from build123d import *

# Parameters (mm, degrees)
F1_DEPTH = 190.5
F2_W     = 260.35
F2_H     = 63.5
F3_DEPTH = 95.25
F4_W     = 31.75
F4_H     = 9.525
F4_R     = 3.175
F5_DEPTH = 76.2


with BuildPart() as f1:
    # F0 (on Right) → F1 (new body, symmetric)
    with BuildSketch(Plane.YZ):
        Polygon((-266.7, 25.4), (-266.7, 0), (0, 0), (0, 304.8), (-9.525, 304.8), (-9.525, 25.4), align=None)
    extrude(amount=F1_DEPTH, both=True)

    # F2 (on face) → F3 (join)
    with BuildSketch(Plane(origin=(0, 0, 0), x_dir=(-1, 0, 0), z_dir=(0, 1, 0))):
        with Locations((0, 31.75)):
            Rectangle(F2_W, F2_H)
    extrude(amount=F3_DEPTH)

    # F4 (on face) → F5 (join)
    with BuildSketch(Plane(origin=(0, 95.25, 0), x_dir=(-1, 0, 0), z_dir=(0, 1, 0))):
        with Locations((15.875, 14.2875)):
            Rectangle(F4_W, F4_H)
        with Locations((73.025, 14.2875)):
            Rectangle(F4_W, F4_H)
        with Locations((15.875, 33.3375)):
            Rectangle(F4_W, F4_H)
        with Locations((44.45, 14.2875)):
            Circle(F4_R)
    extrude(amount=F5_DEPTH)


solid = f1.part
Check sheet for the modelled part. Datum: model origin and axes. Units: mm. A direction names the side the tool comes from. Give positions to 0.01 mm unless a question says otherwise; leave off trailing zeros. Write each loop counter-clockwise with the first axis right and the second up, starting at its lowest first coordinate (ties: lowest second). Pieces come first, ordered by that corner, then holes. Notation, with made-up numbers: (35.5, -14) -> (51.5, -14) arc R14 cw to (51.5, -1) -> close; hole circle Ø7 at (-4.75, 2.5). An arc over 180 degrees is marked (long way). One line per item, written item: value. Start each with the question number.
Item 1: Section check A-A on x = 135.5. Record the cut outline in (y, z) (3 decimals).
Item 2: Section check D-D on z = 103. Record the cut outline in (x, y) (3 decimals).
Item 3: Section check B-B on y = 120. State how many separate pieces and enclosed holes the cut face has, then the cut area to 3 significant figures.
Item 4: Gauge pin test, flat ends, axial feed: pin 1 (12 mm diameter, centred on x = 129, z = 116, fed in from +Y); pin 2 (9.5 mm diameter, centred on x = -18, y = 138.5, fed in from +Z); pin 3 (4 mm diameter, centred on x = -7.5, z = 151, fed in from -Y) (3 decimals). Record the tip position at first contact, or that the pin passes through.
Item 5: Tool access check on faces 1 (the flat face through (130.175, 47, 31)), 2 (the flat face through (-16, 133, 19.05)), 3 (the flat face through (-130.175, 47, 31)), 4 (the flat face through (-73, 133, 19.05)). Record the directions out of +Z, -Z, +X, -X, +Y, -Y that give a thin tool (end or side, any length) a straight path to the whole face; none if there is none.
Item 6: Section check C-C on y = -32. Record the cut outline in (x, z).
Item 7: Material ranges on probe 1 along Z at (x, y) = (83, -48.5); probe 2 along Y at (x, z) = (-94, 129.5) (3 decimals); probe 3 along Z at (x, y) = (87, 21), recorded low to high. Write a range as from..to.
Results list:
1. outline: (-266.7, 0) -> (0, 0) -> (0, 304.8) -> (-9.525, 304.8) -> (-9.525, 25.4) -> (-266.7, 25.4) -> close
2. outline: (-190.5, -9.525) -> (190.5, -9.525) -> (190.5, 0) -> (-190.5, 0) -> close
3. separate pieces: 4
3. enclosed holes: 0
3. area: 939 mm²
4. pin 1: y = 0
4. pin 2: z = 38.1
4. pin 3: y = -9.525
5. face 1: +Z, -Z, +X, +Y
5. face 2: +X, -X, +Y
5. face 3: +Z, -Z, -X, +Y
5. face 4: +Z, +X, -X, +Y
6. outline: (-190.5, 0) -> (190.5, 0) -> (190.5, 25.4) -> (-190.5, 25.4) -> close
7. probe 1: 0..25.4
7. probe 2: -9.525..0
7. probe 3: 0..63.5
